Geometry: final body of the model. Coordinates: model frame, mm. A direction names the side the tool comes from. Give positions to 0.01 mm unless a question says otherwise; leave off trailing zeros. Write each loop counter-clockwise with the first axis right and the second up, starting at its lowest first coordinate (ties: lowest second). Pieces come first, ordered by that corner, then holes. Notation, with made-up numbers: M 84,-28.75 L 88,-28.75 A22 ccw 88,10.25 Z; hole C 6.25,57 d4. An arc over 180 degrees is marked long. Answer as a JSON object with one key per item and string values.
from build123d import *

# Parameters (mm, degrees)
F0_R     = 25
F1_DEPTH = 2
F3_DEPTH = 2.001
F4_R     = 1.25
F5_DEPTH = 2.001
F6_R     = 12.5
F7_DEPTH = 2.001
F8_R     = 3


with BuildPart() as f1:
    # F0 (on Front) → F1 (new body)
    with BuildSketch(Plane.XZ):
        Circle(F0_R)
    extrude(amount=F1_DEPTH)

    # F2 (on face) → F3 (cut, through all)
    with BuildSketch(Plane.XZ.offset(2)):
        with BuildLine():
            Line((-1, 11.3160652761), (-9.3, 6.5240580418))
            ThreePointArc((-9.3, 6.5240580418), (-10.0320508076, 5.7920072343), (-10.3, 4.7920072343))
            Line((-10.3, 4.7920072343), (-10.3, -4.7920072343))
            ThreePointArc((-10.3, -4.7920072343), (-10.0320508076, -5.7920072343), (-9.3, -6.5240580418))
            Line((-9.3, -6.5240580418), (-1, -11.3160652761))
            ThreePointArc((-1, -11.3160652761), (0, -11.5840144685), (1, -11.3160652761))
            Line((1, -11.3160652761), (9.3, -6.5240580418))
            ThreePointArc((9.3, -6.5240580418), (10.0320508076, -5.7920072343), (10.3, -4.7920072343))
            Line((10.3, -4.7920072343), (10.3, 0.3542550839))
            Line((10.3, 0.3542550839), (0, 0.3542550839))
            Line((0, 0.3542550839), (0, 11.5840144685))
            ThreePointArc((0, 11.5840144685), (-0.5176380902, 11.5158661211), (-1, 11.3160652761))
        make_face()
        with BuildLine():
            ThreePointArc((1, 11.3160652761), (0.5176380902, 11.5158661211), (0, 11.5840144685))
            Line((0, 11.5840144685), (0, 0.3542550839))
            Line((0, 0.3542550839), (10.3, 0.3542550839))
            Line((10.3, 0.3542550839), (10.3, 4.7920072343))
            ThreePointArc((10.3, 4.7920072343), (10.0320508076, 5.7920072343), (9.3, 6.5240580418))
            Line((9.3, 6.5240580418), (1, 11.3160652761))
        make_face()
    extrude(amount=-F3_DEPTH, mode=Mode.SUBTRACT)

    # F4 (on face) → F5 (cut, through all)
    with BuildSketch(Plane.XZ.offset(2)):
        with Locations((0, 20)):
            Circle(F4_R)
        with Locations((-17.3205080757, 10)):
            Circle(F4_R)
        with Locations((-17.3205080757, -10)):
            Circle(F4_R)
        with Locations((0, -20)):
            Circle(F4_R)
        with Locations((17.3205080757, -10)):
            Circle(F4_R)
        with Locations((17.3205080757, 10)):
            Circle(F4_R)
    extrude(amount=-F5_DEPTH, mode=Mode.SUBTRACT)

    # F6 (on face) → F7 (cut, through all)
    with BuildSketch(Plane.XZ.offset(2)):
        with BuildLine():
            ThreePointArc((17.5, 0), (30, -12.5), (42.5, 0))
            ThreePointArc((42.5, 0), (30, 12.5), (17.5, 0))
        make_face()
        with BuildLine():
            ThreePointArc((-27.4171924337, 27.4171924337), (-23.8388347648, 17.1419273487), (-13.5635696798, 13.5635696798))
            Line((-13.5635696798, 13.5635696798), (-27.4171924337, 27.4171924337))
        make_face()
        with BuildLine():
            Line((-27.4171924337, 27.4171924337), (-13.5635696798, 13.5635696798))
            ThreePointArc((-13.5635696798, 13.5635696798), (-5.6671178353, 17.6652759282), (-2.5, 25.9807621135))
            ThreePointArc((-2.5, 25.9807621135), (-14.2805924038, 38.4600430508), (-27.4171924337, 27.4171924337))
        make_face()
        with Locations((15, 25.9807621135)):
            Circle(F6_R)
        with Locations((-30, 0)):
            Circle(F6_R)
        with Locations((-15, -25.9807621135)):
            Circle(F6_R)
        with Locations((15, -25.9807621135)):
            Circle(F6_R)
    extrude(amount=-F7_DEPTH, mode=Mode.SUBTRACT)

    # F8
    f8_edges = [f1.edges().sort_by_distance(p)[0] for p in [
        (22.8125, -1, 10.226918),
        (22.8125, -1, -10.226918),
        (20.26302, -1, 14.642746),
        (2.54948, -1, 24.869663),
        (20.26302, -1, -14.642746),
        (2.54948, -1, -24.869663),
        (-2.54948, -1, -24.869663),
        (-20.26302, -1, -14.642746),
        (-22.8125, -1, -10.226918),
        (-22.8125, -1, 10.226918),
        (-20.26302, -1, 14.642746),
        (-2.54948, -1, 24.869663),
    ]]
    fillet(f8_edges, radius=F8_R)


solid = f1.part
1) Cut plane C-C on y = -1.1. Give the number of separate pieces and of enclosed holes in the cut face, and give its area (3 significant figures).
Geometry check:
{"separate pieces": "1", "enclosed holes": "7", "area": "917 mm2"}
2) Cut plane B-B on z = -20. Return loops of the section in (x, y).
Geometry check:
{"outline": "M -4.02,-2 L -1.25,-2 L -1.25,0 L -4.02,0 Z; M 1.25,-2 L 4.02,-2 L 4.02,0 L 1.25,0 Z"}
3) Contact query for flat-ended pins moving along their axis: P1, Ø1, axis at x = 7, z = 18, coming from the -Y side (3 decimals); P2, Ø1, axis at y = -1, z = 2.5, coming from the -X side; P3, Ø1, axis at y = -1, z = -2, coming from the +X side; P4, Ø1, axis at y = -1, z = 18, coming from the +X side. Output: stop coordinate, or through.
Geometry check:
{"P1": "passes through", "P2": "stops at x = -17.87", "P3": "stops at x = 17.75", "P4": "stops at x = 5.82"}
4) Set-up query: faces 5 (the cylindrical face through (-0.015, -1.014, -11.584)), 6 (the cylindrical face through (8.87, -1.014, -15.087)). Return all of +Z, -Z, +X, -X, +Y, -Y with unobstructed straight access to the full face (end or side cutting, diameter ignored); none if empty.
Geometry check:
{"face 5": "+Y, -Y", "face 6": "-Z, +Y, -Y"}
5) Line query: line 1 (Z direction, x = 17, y = -1); line 2 (Z direction, x = -6.5, y = -0.7); line 3 (Z direction, x = -2, y = -0.2). Output: solid intervals per line, ascending. Write a range as from..to.
Geometry check:
{"line 1": "z = -13.64..-11.21, -8.79..8.79, 11.21..13.64", "line 2": "z = -16.82..-8.14, 8.14..16.82", "line 3": "z = -24.25..-10.74, 10.74..24.25"}
6) Cut plane A-A on x = 4.5. Return loops of the section in (y, z).
Geometry check:
{"outline": "M -2,-19.2 L 0,-19.2 L 0,-9.3 L -2,-9.3 Z; M -2,9.3 L 0,9.3 L 0,19.2 L -2,19.2 Z"}
7) Pull-direction query (Z, two-part tool) for faces 1 (the flat face through (-5, 0, 11)), 2 (the flat face through (-5.092, -1.014, 8.954)), 3 (the cylindrical face through (-8.631, -1.014, -15.225)), 4 (the cylindrical face through (8.631, -1.014, 15.225)); classes: pulls with the +Z half, pulls with the -Z half, needs draft (parallel to the pull), parting line crosses it, or undercut.
Geometry check:
{"face 1": "needs draft", "face 2": "undercut", "face 3": "pulls with the -Z half", "face 4": "pulls with the +Z half"}
